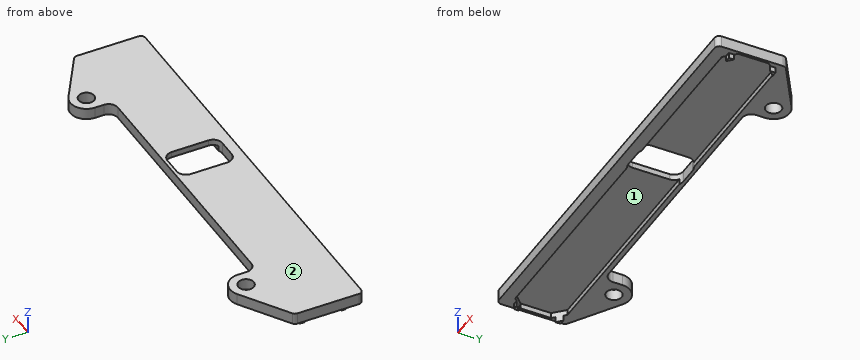
```python
from build123d import *

# Parameters (mm, degrees)
BOSS_EXTRUDE1_DEPTH   = 3.175
F_6_CLEARANCE_HOLE1_D = 4.3053
FILLET3_R             = 1.27
SKETCH4_W             = 10.08
SKETCH4_H             = 15.24
CUT_EXTRUDE1_DEPTH    = 4.175
FILLET4_R             = 2.54
CUT_EXTRUDE2_DEPTH    = 1.524
BOSS_EXTRUDE2_DEPTH   = 1.524


with BuildPart() as part:
    # Sketch1 → Boss-Extrude1 (new body)
    with BuildSketch(Plane.XY):
        with BuildLine():
            Line((58.7375, -67.1354797), (58.7375, -48.0854797))
            Line((58.7375, -48.0854797), (44.939976119, -39.26086832))
            ThreePointArc((44.939976119, -39.26086832), (40.410479427, -39.106525106), (38.1, -43.0054797))
            Line((38.1, -43.0054797), (38.1, -45.5454797))
            ThreePointArc((38.1, -45.5454797), (37.356051224, -47.341530924), (35.56, -48.0854797))
            Line((35.56, -48.0854797), (-35.56, -48.0854797))
            ThreePointArc((-35.56, -48.0854797), (-37.356051224, -47.341530924), (-38.1, -45.5454797))
            Line((-38.1, -45.5454797), (-38.1, -43.0054797))
            ThreePointArc((-38.1, -43.0054797), (-40.410479427, -39.106525106), (-44.939976119, -39.26086832))
            Line((-44.939976119, -39.26086832), (-58.7375, -48.0854797))
            Line((-58.7375, -48.0854797), (-58.7375, -67.1354797))
            Line((-58.7375, -67.1354797), (58.7375, -67.1354797))
        make_face()
    extrude(amount=BOSS_EXTRUDE1_DEPTH)

    # #6 Clearance Hole1 (through all)
    with Locations(Plane(origin=(0, 0, 0), x_dir=(-1, 0, 0), z_dir=(0, 0, -1))):
        with Locations((42.545, -43.0054797), (-42.545, -43.0054797)):
            Hole(F_6_CLEARANCE_HOLE1_D / 2)

    # Fillet3
    fillet3_edges = [part.edges().sort_by_distance(p)[0] for p in [
        (-58.7375, -67.1354797, 1.5875),
        (-58.7375, -48.0854797, 1.5875),
        (58.7375, -48.0854797, 1.5875),
        (58.7375, -67.1354797, 1.5875),
    ]]
    fillet(fillet3_edges, radius=FILLET3_R)

    # Sketch4 → Cut-Extrude1 (cut, through all)
    with BuildSketch(Plane.XY.offset(3.175)):
        with Locations((8.426666963, -56.6198797)):
            Rectangle(SKETCH4_W, SKETCH4_H)
    extrude(amount=-CUT_EXTRUDE1_DEPTH, mode=Mode.SUBTRACT)

    # Fillet4
    fillet4_edges = [part.edges().sort_by_distance(p)[0] for p in [
        (3.386666963, -64.2398797, 1.5875),
        (3.386666963, -48.9998797, 1.5875),
        (13.466666963, -48.9998797, 1.5875),
        (13.466666963, -64.2398797, 1.5875),
    ]]
    fillet(fillet4_edges, radius=FILLET4_R)

    # Sketch7 → Cut-Extrude2 (cut)
    with BuildSketch(Plane(origin=(0, 0, 0), x_dir=(-1, 0, 0), z_dir=(0, 0, -1))):
        Polygon((58.039, -60.872510434), (58.039, -52.367248965), (55.052630735, -49.3808797), (-55.052631243, -49.3808797), (-58.039000508, -52.367248965), (-58.039000508, -60.872510434), (-55.052631243, -63.8588797), (55.052630735, -63.8588797), align=None)
    extrude(amount=-CUT_EXTRUDE2_DEPTH, mode=Mode.SUBTRACT)

    # Sketch5 → Boss-Extrude2 (add)
    with BuildSketch(Plane(origin=(0, 0, 0), x_dir=(-1, 0, 0), z_dir=(0, 0, -1))):
        Polygon((-55.814631243, -50.1428797), (-57.277000508, -50.1428797), (-57.277000508, -51.605248965), align=None)
        Polygon((-55.814631243, -63.0968797), (-57.277000508, -63.0968797), (-57.277000508, -61.634510434), align=None)
        Polygon((57.277, -61.634510434), (57.277, -63.0968797), (55.814630735, -63.0968797), align=None)
        Polygon((55.814630735, -50.1428797), (57.277, -50.1428797), (57.277, -51.605248965), align=None)
    extrude(amount=BOSS_EXTRUDE2_DEPTH)


solid = part.part
```
Geometry: final body of the model. Coordinates: model frame, mm. Face numbers are marked on the shaded views. Coordinates: 2 decimals unless noted, no trailing zeros. Order: outer loops, then holes, each group sorted by start corner. A loop starts at its lowest first (then second) coordinate and runs counter-clockwise, first axis right, second up. Notation, with made-up numbers: (6.5, 48) -> (32.5, 48) arc R15 cw to (32.5, 71) -> close; hole circle Ø4 at (74.25, 88.25). An arc over 180 degrees is marked (long way). Write item = value, one per line.
(1) Cut plane B-B on y = -55. Return loops of the section in (x, z) (1 decimal).
Solved:
outline = (-58.7, 0) -> (-58, 0) -> (-58, 1.5) -> (3.4, 1.5) -> (3.4, 3.2) -> (-58.7, 3.2) -> close; (13.5, 1.5) -> (58, 1.5) -> (58, 0) -> (58.7, 0) -> (58.7, 3.2) -> (13.5, 3.2) -> close
(2) Cut plane C-C on z = -0.8. Return loops of the section in (x, y).
Solved:
outline = (-57.28, -63.1) -> (-55.81, -63.1) -> (-57.28, -61.63) -> close; (-57.28, -51.61) -> (-55.81, -50.14) -> (-57.28, -50.14) -> close; (55.81, -63.1) -> (57.28, -63.1) -> (57.28, -61.63) -> close; (55.81, -50.14) -> (57.28, -51.61) -> (57.28, -50.14) -> close
(3) Pin query (flat end, axial travel): pin 1 Ø1.2 at (x, z) = (-56.5, -1) entering from +Y; pin 2 Ø1.3 at (y, z) = (-44.5, 1.5) entering from +X; pin 3 Ø8.5 at (x, y) = (27.5, -57.5) entering from -Z. Return the tip coordinate at first contact, or that it passes through.
Solved:
pin_1 = -50.14
pin_2 = 54.15
pin_3 = 1.52
(4) Line query: line 1 (Y direction, x = 19, z = 0.15); line 2 (X direction, y = -60.5, z = 2.7); line 3 (Y direction, x = -34, z = 2.9). Output: solid intervals per line, ascending.
Solved:
line_1 = -67.14 to -63.86, -49.38 to -48.09
line_2 = -58.74 to 3.39, 13.47 to 58.74
line_3 = -67.14 to -48.09
(5) Cut plane D-D on y = -44. Return loops of the section in (x, z) (3 decimals), plus the area to 3 significant figures.
Solved:
outline = (-52.35, 0) -> (-44.454, 0) -> (-44.454, 3.175) -> (-52.35, 3.175) -> close; (-40.636, 0) -> (-38.1, 0) -> (-38.1, 3.175) -> (-40.636, 3.175) -> close; (38.1, 0) -> (40.636, 0) -> (40.636, 3.175) -> (38.1, 3.175) -> close; (44.454, 0) -> (52.35, 0) -> (52.35, 3.175) -> (44.454, 3.175) -> close
area = 66.2 mm²
(6) Pull-direction query (Y, two-part tool) for the marked faces 1 and 2; classes: pulls with the +Y half, pulls with the -Y half, needs draft (parallel to the pull), parting line crosses it, or undercut.
Solved:
face_1 = undercut
face_2 = needs draft
(7) Cut plane A-A on x = 7. Return loops of the section in (y, z) (3 decimals).
Solved:
outline = (-67.135, 0) -> (-64.24, 0) -> (-64.24, 3.175) -> (-67.135, 3.175) -> close; (-49, 0) -> (-48.085, 0) -> (-48.085, 3.175) -> (-49, 3.175) -> close
